Could you check a few things on this drawing? It's one solid part, dimensions in mm from its lowest x, y, z. A direction names the side the tool comes from. Round coordinates to 2 decimals unless told otherwise and drop trailing zeros. Loops run counter-clockwise (first coordinate to the right, second up) from the corner with the lowest first, then second, coordinate; pieces in that order, holes last.
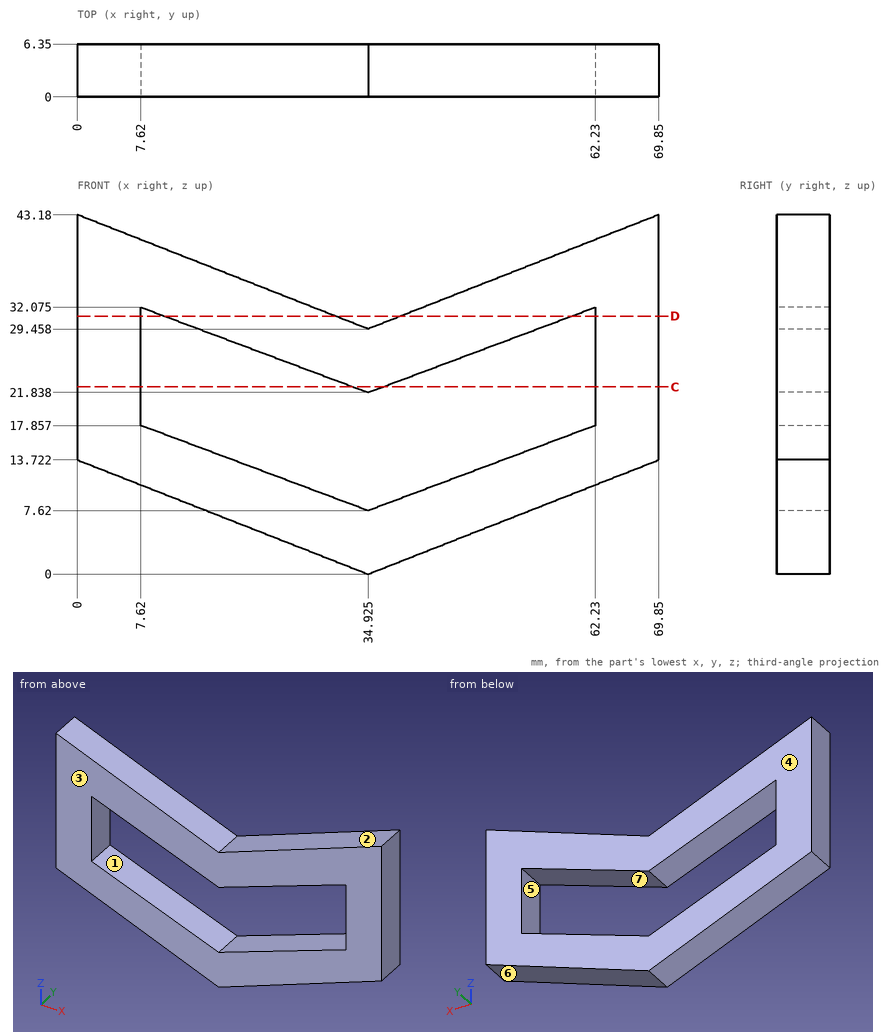
(1) Suppose I cut it at D-D (z = 31). Write out the boundary of the cut face in (x, y).
(2) If I drill on line 1 (Z direction, x = 45.5, y = 1.25) (1 decimal); line 2 (Z direction, x = 35, y = 0.5) (1 decimal); line 3 (Z direction, x = 63, y = 4), over which ranges is the centre line in solid material (lowest first)?
(3) We'd pull the mould along X, two halves only. Please class the marked faces 4, 5, 6 and 7: released by +X, released by -X, zero draft, split by the parting line, or undercut.
(4) Suppose I cut it at C-C (z = 22.5). Write out the boundary of the cut face in (x, y).
(5) For pin 1 (8 mm diameter, centred on x = 18, z = 9, fed in from -Y), with a flat end and sliding along its axis, tell me the tip position at first contact or that it passes through.
(6) Which directions (+Z, -Z, +X, -X, +Y, -Y) give clear straight access to the entire face, cutting with the end or side of a thin tool? Please do the marked faces 1, 2 and 3.
Check result:
1. outline: (0, 0) - (7.62, 0) - (7.62, 6.35) - (0, 6.35) - close; (10.49, 0) - (31, 0) - (31, 6.35) - (10.49, 6.35) - close; (38.85, 0) - (59.36, 0) - (59.36, 6.35) - (38.85, 6.35) - close; (62.23, 0) - (69.85, 0) - (69.85, 6.35) - (62.23, 6.35) - close
2. line 1: z = 4.2 to 11.6, 25.8 to 33.6
2. line 2: z = 0 to 7.6, 21.9 to 29.5
2. line 3: z = 11.03 to 40.49
3. face 4: zero draft
3. face 5: undercut
3. face 6: released by +X
3. face 7: undercut
4. outline: (0, 0) - (7.62, 0) - (7.62, 6.35) - (0, 6.35) - close; (33.16, 0) - (36.69, 0) - (36.69, 6.35) - (33.16, 6.35) - close; (62.23, 0) - (69.85, 0) - (69.85, 6.35) - (62.23, 6.35) - close
5. pin 1: stops at y = 0
6. face 1: +Y, -Y
6. face 2: +Z, +Y, -Y
6. face 3: +Z, -Z, +X, -X, -Y
